Design review of the part built by this model. Coordinates are the model's own, in mm. A direction names the side the tool comes from. Coordinates: 2 decimals unless noted, no trailing zeros. Loops run counter-clockwise (first coordinate to the right, second up) from the corner with the lowest first, then second, coordinate; pieces in that order, holes last. Notation, with made-up numbers: M -3.75,47.5 L 9.25,47.5 A22 cw 9.25,84.5 Z; hole C 60,10 d5. An arc over 180 degrees is marked long. Put each result on its own line as item: value. Start each with the question number.
(1) Take a section at B-B, the plane z = 0. Give the boundary of the cut face in (x, y), then the cut area to 3 significant figures.
(2) Clearance check with flat-ended pins moving along their axes: pin 1 (8 mm diameter, centred on x = 35, z = 13, fed in from -Y); pin 2 (4 mm diameter, centred on x = 38, z = -5, fed in from -Y); pin 3 (12 mm diameter, centred on x = 25, z = -12, fed in from -Y). State where each tip first meets the part, or that it passes through.
(3) For probe 1 along Z at (x, y) = (21, 0); probe 2 along X at (y, z) = (-11.5, -11); probe 3 along Z at (x, y) = (11.5, 1), list the stretches that pass through material, from the lowest coordinate up. Write a range as [from, to].
(4) For faces 5 (the cylindrical face through (2, 0, -20)), 6 (the cylindrical face through (25.952, -0.66, -14.985)), list the 3-axis set-ups (+Z, -Z, +X, -X, +Y, -Y) from which the entire face can be reached by the end or side of a thin tool; tool diameter is ignored.
(5) Take a section at D-D, the plane z = 16.5. Give the boundary of the cut face in (x, y).
(6) The part is to be moulded in two halves that separate along Z. For faces 1 (the cylindrical face through (29.58, 1.08, -4.88)), 2 (the cylindrical face through (2, 0, 20)), 3 (the flat face through (5, 13, 8)), 4 (the cylindrical face through (55.704, -0.66, -14.985)), say which applies: +Z half, -Z half, draft (parallel to the pull), parting line (faces both ways), or undercut.
(7) Take a section at C-C, the plane x = 18.5. Give the boundary of the cut face in (y, z).
(8) Take a section at A-A, the plane y = 0. Give the boundary of the cut face in (x, z).
```python
from build123d import *

# Parameters (mm, degrees)
F3_SIZE  = 1
F1_R     = 2.5
F6_DEPTH = 5
F7_R     = 5
F8_DEPTH = 60


with BuildPart() as f2:
    # F0 (on Front) → F2 (revolve)
    with BuildSketch(Plane.XZ):
        Polygon((0, 20), (0, 0), (60, 0), (60, 15), (5, 15), (5, 20), align=None)
    revolve(axis=Axis((30, 0, 0), (1, 0, 0)))

    # F3
    f3_edges = [f2.edges().sort_by_distance(p)[0] for p in [
        (60, 0, -15),
    ]]
    chamfer(f3_edges, length=F3_SIZE)

    # F1 (on face) → F4 (revolve, cut)
    with BuildSketch(Plane.XZ):
        with Locations((50, 15)):
            Circle(F1_R)
    revolve(axis=Axis((30, 0, 0), (1, 0, 0)), mode=Mode.SUBTRACT)

    # F5 (on face) → F6 (cut, through all)
    with BuildSketch(Plane(origin=(0, 0, 0), x_dir=(0, -1, 0), z_dir=(-1, 0, 0))):
        with BuildLine():
            Line((18, 8.7177978871), (18, -8.7177978871))
            ThreePointArc((18, -8.7177978871), (19.4935886896, -4.472135955), (20, 0))
            ThreePointArc((20, 0), (19.4935886896, 4.472135955), (18, 8.7177978871))
        make_face()
        with BuildLine():
            ThreePointArc((-18, 8.7177978871), (-20, 0), (-18, -8.7177978871))
            Line((-18, -8.7177978871), (-18, 8.7177978871))
        make_face()
    extrude(amount=-F6_DEPTH, mode=Mode.SUBTRACT)

    # F7 (on face) → F8 (cut, through all)
    with BuildSketch(Plane(origin=(0, 0, 0), x_dir=(0, -1, 0), z_dir=(-1, 0, 0))):
        Circle(F7_R)
    extrude(amount=-F8_DEPTH, mode=Mode.SUBTRACT)


solid = f2.part
```
Computed values:
1. outline: M 0,-18 L 5,-18 L 5,-15 L 47.5,-15 A2.5 cw 52.5,-15 L 59,-15 L 60,-14 L 60,-5 L 0,-5 Z; M 0,5 L 60,5 L 60,14 L 59,15 L 52.5,15 A2.5 cw 47.5,15 L 5,15 L 5,18 L 0,18 Z
1. area: 1,210 mm^2
2. pin 1: stops at y = -12
2. pin 2: stops at y = -14.7
2. pin 3: stops at y = -13.75
3. probe 1: z = [-15, -5], [5, 15]
3. probe 2: x = [0, 5]
3. probe 3: z = [-14.97, -4.9], [4.9, 14.97]
4. face 5: -Z, +X, -X
4. face 6: +X
5. outline: M 0,-11.3 L 5,-11.3 L 5,11.3 L 0,11.3 Z
6. face 1: undercut
6. face 2: +Z half
6. face 3: draft
6. face 4: parting line
7. outline: C 0,0 d30; hole C 0,0 d10
8. outline: M 0,-20 L 5,-20 L 5,-15 L 47.5,-15 A2.5 cw 52.5,-15 L 59,-15 L 60,-14 L 60,-5 L 0,-5 Z; M 0,5 L 60,5 L 60,14 L 59,15 L 52.5,15 A2.5 cw 47.5,15 L 5,15 L 5,20 L 0,20 Z
